For this review, take the finished solid that the model builds, in its own axes (mm). Face numbers are marked on the shaded views. Round coordinates to 2 decimals unless told otherwise and drop trailing zeros. Order: outer loops, then holes, each group sorted by start corner. A loop starts at its lowest first (then second) coordinate and runs counter-clockwise, first axis right, second up. Notation, with made-up numbers: M 87.5,-9.75 L 113.5,-9.75 A28 ccw 113.5,9.25 Z; hole C 70.25,3.5 d9. An arc over 180 degrees is marked long. Answer as a JSON object with one key per item and string values.
from build123d import *

# Parameters (mm, degrees)
F0_R          = 14.187969
F0_R_2        = 7.743586
F1_DEPTH      = 27.278503
F4_DEPTH      = 70.82668
F4_DEPTH_BACK = 25.4
F5_R          = 0.2032


with BuildPart() as f1:
    # F0 (on Top) → F1 (new body)
    with BuildSketch(Plane.XY):
        with BuildLine():
            ThreePointArc((-23.337792, 3.076938), (0, 23.539755), (23.337792, 3.076938))
            Line((23.337792, 3.076938), (15.189044, 64.883116))
            ThreePointArc((15.189044, 64.883116), (15.287592, 63.883982), (15.320488, 62.880538))
            ThreePointArc((15.320488, 62.880538), (-1.003444, 47.592947), (-15.189044, 64.883116))
            Line((-15.189044, 64.883116), (-23.337792, 3.076938))
        make_face()
        with BuildLine():
            ThreePointArc((-23.337792, 3.076938), (-1.54178, -23.48921), (23.539755, 0))
            ThreePointArc((23.539755, 0), (23.48921, 1.54178), (23.337792, 3.076938))
            ThreePointArc((23.337792, 3.076938), (0, 23.539755), (-23.337792, 3.076938))
        make_face()
        Circle(F0_R, mode=Mode.SUBTRACT)
        with BuildLine():
            ThreePointArc((15.320488, 62.880538), (15.287592, 63.883982), (15.189044, 64.883116))
            ThreePointArc((15.189044, 64.883116), (0, 78.201027), (-15.189044, 64.883116))
            ThreePointArc((-15.189044, 64.883116), (-1.003444, 47.592947), (15.320488, 62.880538))
        make_face()
        with Locations((0, 62.880538)):
            Circle(F0_R_2, mode=Mode.SUBTRACT)
    extrude(amount=F1_DEPTH)

    # F3 (on Right) → F4 (cut, two sides)
    with BuildSketch(Plane.YZ) as f4_sk:
        Polygon((98.717824, 27.551521), (12.098692, 27.551521), (98.717824, 7.182653), align=None)
    extrude(amount=F4_DEPTH, mode=Mode.SUBTRACT)
    extrude(f4_sk.sketch, amount=-F4_DEPTH_BACK, mode=Mode.SUBTRACT)

    # F5
    f5_edges = [f1.edges().sort_by_distance(p)[0] for p in [
        (-8.052412, -11.681487, 27.278503),
        (-1.54178, -23.48921, 27.278503),
        (18.592151, 39.071411, 21.208768),
        (-13.521451, 13.259705, 27.278503),
        (13.521451, 13.259705, 27.278503),
    ]]
    fillet(f5_edges, radius=F5_R)


solid = f1.part
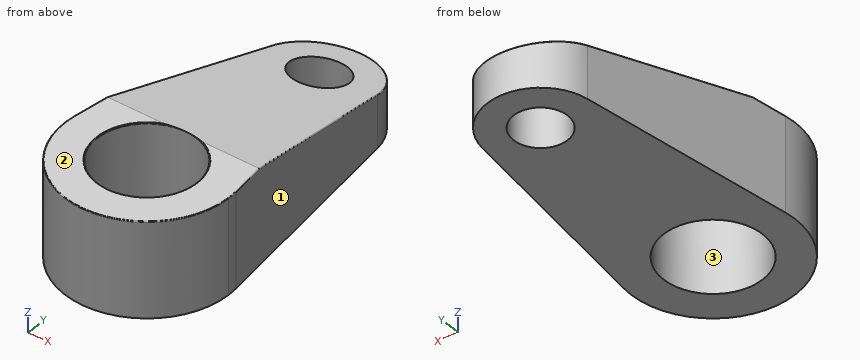
1) Add section A-A on z = 9.5. State the section outline as (x, y) points, and give its area (3 significant figures).
Geometry check:
{"outline": "M -23.34,3.08 A23.54 ccw long 23.54,0 A23.54 ccw 23.34,3.08 L 15.19,64.88 A15.32 ccw -15.19,64.88 Z; hole C 0,0 d28.38; hole C 0,62.88 d15.49", "area": "2,880 mm²"}
2) Add section B-B on x = 0. State how many separate pieces and enclosed holes the cut face has, and give its area (3 significant figures).
Geometry check:
{"separate pieces": "3", "enclosed holes": "0", "area": "1,260 mm²"}
3) For L1, parallel to Y at x = 0, z = 9; L2, parallel to X at y = 0, z = 6.25; L3, parallel to Y at x = 6, z = 4.25, list the stretches that pass through material, from the lowest coordinate up.
Geometry check:
{"L1": "y = -23.54 to -14.19, 14.19 to 55.14, 70.62 to 78.2", "L2": "x = -23.54 to -14.19, 14.19 to 23.54", "L3": "y = -22.76 to -12.86, 12.86 to 57.99, 67.78 to 76.98"}
4) Insertion check: P1, Ø12, axis at y = 47, z = 12.5, coming from the +X side; P2, Ø2, axis at y = -11.5, z = 5.5, coming from the -X side; P3, Ø3, axis at x = -11, z = 8.5, coming from the -Y side; P4, Ø14, axis at x = 0, y = 62.88, coming from the +Z side. Each pin has a flat end and moves straight along its axis. Give the tip position at first contact, or say it passes through.
Geometry check:
{"P1": "stops at x = 18.34", "P2": "stops at x = -21.07", "P3": "stops at y = -21.54", "P4": "passes through"}
5) Mouldability with a two-part tool opening along X and no side actions: class the marked faces 1, 2 and 3 as +X half, -X half, draft (parallel to the pull), parting line (faces both ways), or undercut.
Geometry check:
{"face 1": "+X half", "face 2": "draft", "face 3": "undercut"}
